Verification items for the finished model (mm, model axes). A direction names the side the tool comes from. Give positions to 0.01 mm unless a question says otherwise; leave off trailing zeros. Write each loop counter-clockwise with the first axis right and the second up, starting at its lowest first coordinate (ties: lowest second). Pieces come first, ordered by that corner, then holes. Notation, with made-up numbers: (31, 59.25) - (90, 59.25) arc R20 cw to (90, 82.25) - close; hole circle Ø10 at (8.25, -5.75). An arc over 180 degrees is marked (long way). Put each result on its own line as item: value.
from build123d import *

# Parameters (mm, degrees)
BOSS_EXTRUDE1_DEPTH = 6
SKETCH2_R           = 6
BOSS_EXTRUDE2_DEPTH = 12
SKETCH3_R           = 3
CUT_EXTRUDE1_DEPTH  = 12
SKETCH4_R           = 1.5
CUT_EXTRUDE2_DEPTH  = 21.375127811


with BuildPart() as part:
    # Sketch1 → Boss-Extrude1 (new body)
    with BuildSketch(Plane(origin=(0, 0, 0), x_dir=(0, 0, -1), z_dir=(1, 0, 0))):
        Polygon((7.216878365, 0), (3.608439182, 6.25), (-3.608439182, 6.25), (-7.216878365, 0), (-3.608439182, -6.25), (3.608439182, -6.25), align=None)
    extrude(amount=BOSS_EXTRUDE1_DEPTH)

    # Sketch2 → Boss-Extrude2 (add)
    with BuildSketch(Plane.ZY):
        with Locations(Location((0, 0, 0), (0, 0, 180))):
            Circle(SKETCH2_R)
    extrude(amount=BOSS_EXTRUDE2_DEPTH)

    # Sketch3 → Cut-Extrude1 (cut)
    with BuildSketch(Plane.ZY.offset(12)):
        Circle(SKETCH3_R)
    extrude(amount=-CUT_EXTRUDE1_DEPTH, mode=Mode.SUBTRACT)

    # Sketch4 → Cut-Extrude2 (cut, through all)
    with BuildSketch(Plane(origin=(6, 0, 0), x_dir=(0, 0, -1), z_dir=(1, 0, 0))):
        Circle(SKETCH4_R)
    extrude(amount=-CUT_EXTRUDE2_DEPTH, mode=Mode.SUBTRACT)


solid = part.part
Q1. Release check for a two-part mould opening along Z. For faces 3 (the face through (0, -1.3, 1.3)), 4 (the face through (-12, 1, 3)), 5 (the face through (2.96, 3.08, -5.44)), 6 (the face through (2.958, 3.169, 5.387)) record: released by +Z, released by -Z, zero draft, split by the parting line, or undercut.
Answers follow:
face 3: undercut
face 4: zero draft
face 5: released by -Z
face 6: released by +Z
Q2. Section check D-D, the plane y = 4.75. Record the cut outline in (x, z).
Answers follow:
outline: (-12, -3.67) - (0, -3.67) - (0, -4.47) - (6, -4.47) - (6, 4.47) - (0, 4.47) - (0, 3.67) - (-12, 3.67) - close
Q3. Scan lines: line 1 along Y through (x, z) = (-8.25, 0); line 2 along Y through (x, z) = (2, 0); line 3 along Z through (x, y) = (-4, -1.5). Record each from-to range of solid material in increasing order.
Answers follow:
line 1: y = -6 to -3, 3 to 6
line 2: y = -6.25 to -1.5, 1.5 to 6.25
line 3: z = -5.81 to -2.6, 2.6 to 5.81
Q4. Go/stop test with flat-tipped pins: pin 1 Ø1.5 at (x, y) = (-4.5, -1.5) entering from +Z; pin 2 Ø5 at (x, y) = (-7, -4) entering from -Z; pin 3 Ø5 at (x, y) = (4, -5) entering from +Z. Record where each tip stops, or that it passes through.
Answers follow:
pin 1: stops at z = 5.95
pin 2: stops at z = -5.81
pin 3: stops at z = 5.77
Q5. Section check C-C, the plane y = 0.25. Record the cut outline in (x, z), plus the area to 3 significant figures.
Answers follow:
outline: (-12, -5.99) - (0, -5.99) - (0, -7.07) - (6, -7.07) - (6, -1.48) - (0, -1.48) - (0, -2.99) - (-12, -2.99) - close; (-12, 2.99) - (0, 2.99) - (0, 1.48) - (6, 1.48) - (6, 7.07) - (0, 7.07) - (0, 5.99) - (-12, 5.99) - close
area: 139 mm2
Q6. Section check A-A, the plane z = 0. Record the cut outline in (x, y), plus the area to 3 significant figures.
Answers follow:
outline: (-12, -6) - (0, -6) - (0, -6.25) - (6, -6.25) - (6, -1.5) - (0, -1.5) - (0, -3) - (-12, -3) - close; (-12, 3) - (0, 3) - (0, 1.5) - (6, 1.5) - (6, 6.25) - (0, 6.25) - (0, 6) - (-12, 6) - close
area: 129 mm2
Q7. Section check B-B, the plane x = 4.75. Record the cut outline in (y, z), plus the area to 3 significant figures.
Answers follow:
outline: (-6.25, -3.61) - (0, -7.22) - (6.25, -3.61) - (6.25, 3.61) - (0, 7.22) - (-6.25, 3.61) - close; hole circle Ø3 at (0, 0)
area: 128 mm2
Q8. Set-up check for faces 1 (the face through (2.958, -3.169, -5.387)), 2 (the face through (-6, 0, -3)): record each of +Z, -Z, +X, -X, +Y, -Y from which the full face is reachable in a straight line by a thin tool's end or side.
Answers follow:
face 1: -Z, +X, -X, -Y
face 2: -X
